Verification items for this drawing (mm, ordinates from the low corner). A direction names the side the tool comes from. Give positions to 0.01 mm unless a question says otherwise; leave off trailing zeros. Write each loop counter-clockwise with the first axis right and the second up, starting at its lowest first coordinate (ties: lowest second). Pieces come first, ordered by that corner, then holes. Notation, with made-up numbers: (34, 14) -> (48, 14) arc R24 cw to (48, 39) -> close; hole circle Ø2 at (68, 54). An arc over 180 degrees is marked (long way). Answer as a JSON object with one key per item and string values.
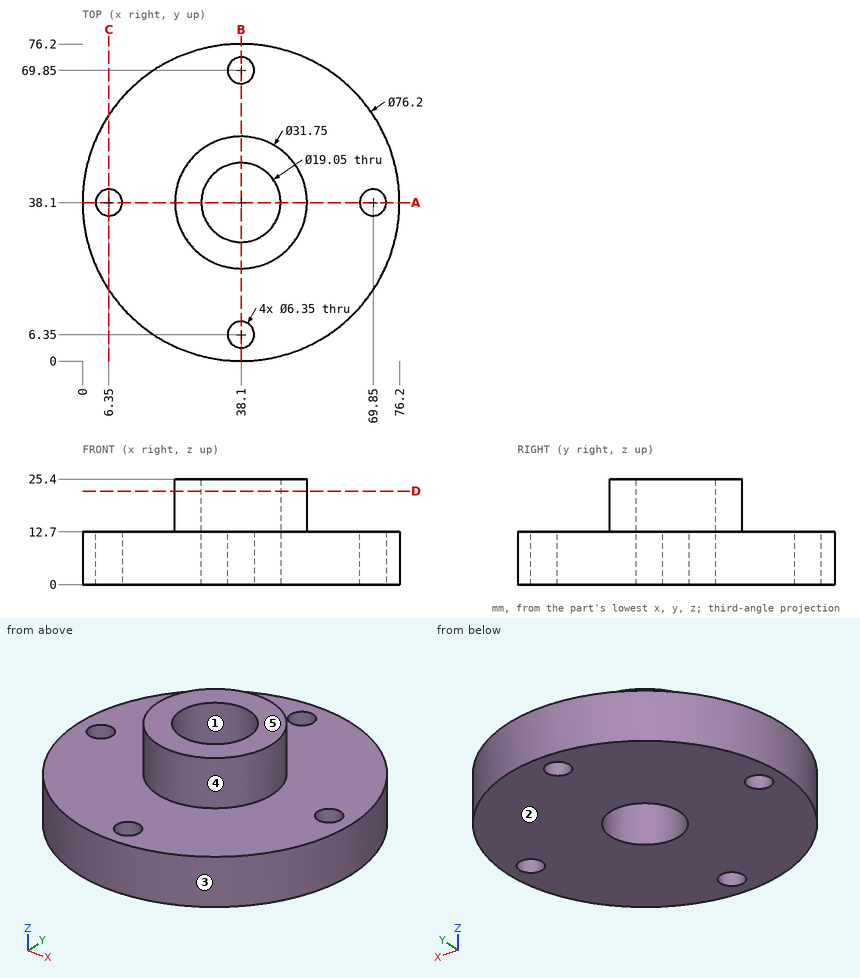
1. Go/stop test with flat-tipped pins: P1, Ø1, axis at y = 38.5, z = 15.5, coming from the -X side (3 decimals); P2, Ø1.5, axis at x = 49, z = 18, coming from the -Y side; P3, Ø5.5, axis at x = 69.85, y = 38.1, coming from the -Z side; P4, Ø10, axis at y = 40.5, z = 13, coming from the +X side. Record where each tip stops, or that it passes through.
Determined:
{"P1": "x = 22.225", "P2": "y = 25.89", "P3": "through", "P4": "x = 76.2"}
2. Sectioned sample at A-A, the plane y = 38.1. Enter the section's corners in (x, z) (3 decimals), plus the area to 3 significant figures.
Determined:
{"outline": "(0, 0) -> (3.175, 0) -> (3.175, 12.7) -> (0, 12.7) -> close; (9.525, 0) -> (28.575, 0) -> (28.575, 25.4) -> (22.225, 25.4) -> (22.225, 12.7) -> (9.525, 12.7) -> close; (47.625, 0) -> (66.675, 0) -> (66.675, 12.7) -> (53.975, 12.7) -> (53.975, 25.4) -> (47.625, 25.4) -> close; (73.025, 0) -> (76.2, 0) -> (76.2, 12.7) -> (73.025, 12.7) -> close", "area": "726 mm^2"}
3. Sectioned sample at D-D, the plane z = 22.5. Enter the section's corners in (x, y) (3 decimals).
Determined:
{"outline": "circle Ø31.75 at (38.1, 38.1); hole circle Ø19.05 at (38.1, 38.1)"}
4. Sectioned sample at C-C, the plane x = 6.35. Enter the section's corners in (y, z) (3 decimals).
Determined:
{"outline": "(17.039, 0) -> (34.925, 0) -> (34.925, 12.7) -> (17.039, 12.7) -> close; (41.275, 0) -> (59.161, 0) -> (59.161, 12.7) -> (41.275, 12.7) -> close"}
5. Mould release check, pull along Y, two halves, no side actions. Record for the marked faces 1, 2 and 3: released by +Y, released by -Y, zero draft, split by the parting line, or undercut.
Determined:
{"face 1": "undercut", "face 2": "zero draft", "face 3": "split by the parting line"}
6. Scan lines: L1, parallel to Y at x = 38.1, z = 2.75 (3 decimals); L2, parallel to Y at x = 38.1, z = 16 (3 decimals); L3, parallel to Z at x = 67, y = 60. Record each from-to range of solid material in increasing order. Write a range as [from, to].
Determined:
{"L1": "[0, 3.175], [9.525, 28.575], [47.625, 66.675], [73.025, 76.2]", "L2": "[22.225, 28.575], [47.625, 53.975]", "L3": "[0, 12.7]"}
7. Access from +Z, -Z, +X, -X, +Y, -Y to the whole of each face (thin tool, end or side, straight path). Record for the marked faces 4 and 5.
Determined:
{"face 4": "+Z", "face 5": "+Z, +X, -X, +Y, -Y"}
